```python
from build123d import *

# Parameters (mm, degrees)
F0_R        = 2
F1_DEPTH    = 3.175
F2_R        = 5
F3_R        = 2
F4_W        = 3
F4_H        = 26
F5_DEPTH    = 1
F6_T1_DEPTH = 26


# Not quite as in the source:
# - a fillet or chamfer that OpenCascade refuses, or shapes differently, is made with other operations: its cross-section is extruded or revolved along the edge and cut away or added


with BuildPart() as f1:
    # F0 (on Top) → F1 (new body)
    with BuildSketch(Plane.XY):
        with BuildLine():
            Line((11.2449979984, 0), (0, 0))
            Line((0, 0), (0, 11.2449979984))
            ThreePointArc((0, 11.2449979984), (-0.6568542495, -0.6568542495), (11.2449979984, 0))
        make_face()
        Polygon((0, 11.2449979984), (0, 0), (11.2449979984, 0), (41, 0), (70.7550020016, 0), (82, 0), (82, 11.2449979984), (82, 26), (57.1, 26), (57.1, 21), (41, 21), (24.9, 21), (24.9, 26), (0, 26), align=None)
        with Locations((5, 5)):
            Circle(F0_R, mode=Mode.SUBTRACT)
        with Locations((77, 5)):
            Circle(F0_R, mode=Mode.SUBTRACT)
        with BuildLine():
            Line((82, 0), (70.7550020016, 0))
            ThreePointArc((70.7550020016, 0), (82.6568542495, -0.6568542495), (82, 11.2449979984))
            Line((82, 11.2449979984), (82, 0))
        make_face()
    extrude(amount=F1_DEPTH)

    # F2
    f2_edges = [f1.edges().sort_by_distance(p)[0] for p in [
        (11.244998, 0, 1.5875),
        (70.755002, 0, 1.5875),
        (82, 11.244998, 1.5875),
        (0, 11.244998, 1.5875),
    ]]
    fillet(f2_edges, radius=F2_R)

    # F3
    f3_edges = [f1.edges().sort_by_distance(p)[0] for p in [
        (24.9, 21, 1.5875),
        (57.1, 21, 1.5875),
    ]]
    fillet(f3_edges, radius=F3_R)

    # F4 (on face) → F5 (join)
    with BuildSketch(Plane.XY.offset(3.175)):
        with Locations((20.4, 13)):
            Rectangle(F4_W, F4_H)
        with Locations((61.6, 13)):
            Rectangle(F4_W, F4_H)
    extrude(amount=F5_DEPTH)

    # F6: fillet of radius 5 on 4 edges, made by hand

    # F6_s2 → F6_t1 (join)
    with BuildSketch(Plane.XZ.offset(-26)):
        with BuildLine():
            ThreePointArc((15.9, 3.175), (17.4811388301, 3.4315835097), (18.9, 4.175))
            Line((18.9, 4.175), (18.96, 4.095))
            ThreePointArc((18.96, 4.095), (19, 3.675), (19, 3.175))
            Line((19, 3.175), (18.9, 3.075))
            Line((18.9, 3.075), (15.9, 3.075))
            Line((15.9, 3.075), (15.9, 3.175))
        make_face()
        with BuildLine():
            ThreePointArc((24.9, 3.175), (23.3188611699, 3.4315835097), (21.9, 4.175))
            Line((21.9, 4.175), (21.84, 4.095))
            ThreePointArc((21.84, 4.095), (21.8, 3.675), (21.8, 3.175))
            Line((21.8, 3.175), (21.9, 3.075))
            Line((21.9, 3.075), (24.9, 3.075))
            Line((24.9, 3.075), (24.9, 3.175))
        make_face()
        with BuildLine():
            ThreePointArc((57.1, 3.175), (58.6811388301, 3.4315835097), (60.1, 4.175))
            Line((60.1, 4.175), (60.16, 4.095))
            ThreePointArc((60.16, 4.095), (60.2, 3.675), (60.2, 3.175))
            Line((60.2, 3.175), (60.1, 3.075))
            Line((60.1, 3.075), (57.1, 3.075))
            Line((57.1, 3.075), (57.1, 3.175))
        make_face()
        with BuildLine():
            ThreePointArc((66.1, 3.175), (64.5188611699, 3.4315835097), (63.1, 4.175))
            Line((63.1, 4.175), (63.04, 4.095))
            ThreePointArc((63.04, 4.095), (63, 3.675), (63, 3.175))
            Line((63, 3.175), (63.1, 3.075))
            Line((63.1, 3.075), (66.1, 3.075))
            Line((66.1, 3.075), (66.1, 3.175))
        make_face()
    extrude(amount=F6_T1_DEPTH)


solid = f1.part
```
Input: part model. Units: mm. Frame: model coordinates. A direction names the side the tool comes from. Round coordinates to 2 decimals unless told otherwise and drop trailing zeros. Order: outer loops, then holes, each group sorted by start corner. A loop starts at its lowest first (then second) coordinate and runs counter-clockwise, first axis right, second up. Notation, with made-up numbers: (53.25, 33.5) - (77.25, 33.5) arc R24 ccw to (77.25, 51.5) - close; hole circle Ø6 at (17, 57.25). An arc over 180 degrees is marked (long way). Answer in a Markdown table with one row per item.
Item 1: Line query: line 1 (X direction, y = 24.5, z = 2.7); line 2 (X direction, y = 3.75, z = 2.8); line 3 (Y direction, x = 77, z = 1.35). Output: solid intervals per line, ascending.
Model answer:
| item | result |
|---|---|
| line 1 | x = 0 to 24.9, 57.1 to 82 |
| line 2 | x = -2.9 to 3.44, 6.56 to 75.44, 78.56 to 84.9 |
| line 3 | y = -3 to 3, 7 to 26 |
Item 2: Section query B-B (z = 1.1). Return the cut outline in (x, y).
Model answer:
| item | result |
|---|---|
| outline | (-1.15, 10.11) arc R8 ccw to (10.11, -1.15) arc R5 cw to (13.31, 0) - (68.69, 0) arc R5 cw to (71.89, -1.15) arc R8 ccw to (83.15, 10.11) arc R5 cw to (82, 13.31) - (82, 26) - (57.1, 26) - (57.1, 23) arc R2 cw to (55.1, 21) - (26.9, 21) arc R2 cw to (24.9, 23) - (24.9, 26) - (0, 26) - (0, 13.31) arc R5 cw to start; hole circle Ø4 at (5, 5); hole circle Ø4 at (77, 5) |
Item 3: Mould query, pull axis X, two halves, no side actions, for faces 6 (the flat face through (75, 12, 3.175)), 7 (the cylindrical face through (64.54, 13.182, 3.425)), 8 (the flat face through (41, 9, 3.175)). Classes: released by +X, released by -X, zero draft, split by the parting line, or undercut.
Model answer:
| item | result |
|---|---|
| face 6 | zero draft |
| face 7 | released by +X |
| face 8 | undercut |
Item 4: Reachability of faces 1 (the flat face through (6, 12, 3.175)), 2 (the cylindrical face through (25.47, 21.6, 1.61)), 3 (the cylindrical face through (70.4, -0.3, 1.6)), 4 (the flat face through (0, 20, 2)), 5 (the cylindrical face through (82.54, -0.77, 1.57)) from +Z, -Z, +X, -X, +Y, -Y: full face, straight path, thin tool, end or side. Return the list, or none.
Model answer:
| item | result |
|---|---|
| face 1 | +Z, -X, +Y, -Y |
| face 2 | +Z, -Z, +Y |
| face 3 | +Z, -Z, -Y |
| face 4 | +Z, -Z, -X, +Y |
| face 5 | +Z, -Z |
Item 5: Section query C-C (y = 20.25). Return the cut outline in (x, z) (3 decimals), then the cut area to 3 significant figures.
Model answer:
| item | result |
|---|---|
| outline | (0, 0) - (82, 0) - (82, 3.175) - (66.1, 3.175) arc R5 cw to (63.1, 4.175) - (60.1, 4.175) arc R5 cw to (57.1, 3.175) - (24.9, 3.175) arc R5 cw to (21.9, 4.175) - (18.9, 4.175) arc R5 cw to (15.9, 3.175) - (0, 3.175) - close |
| area | 270 mm² |
Item 6: Section query A-A (x = 77). Return the cut outline in (y, z) (3 decimals), then the cut area to 3 significant figures.
Model answer:
| item | result |
|---|---|
| outline | (-3, 0) - (3, 0) - (3, 3.175) - (-3, 3.175) - close; (7, 0) - (26, 0) - (26, 3.175) - (7, 3.175) - close |
| area | 79.4 mm² |
Item 7: Pin query (flat end, axial travel): pin 1 (1.6 mm diameter, centred on y = 19.5, z = 1, fed in from -X); pin 2 (2.5 mm diameter, centred on x = 77, y = 5, fed in from +Z); pin 3 (1.5 mm diameter, centred on y = 10.5, z = 1.5, fed in from +X); pin 4 (5.5 mm diameter, centred on x = 8, y = 13.5, fed in from +Z) (3 decimals). Return the tip coordinate at first contact, or that it passes through.
Model answer:
| item | result |
|---|---|
| pin 1 | stops at x = 0 |
| pin 2 | passes through |
| pin 3 | stops at x = 83.44 |
| pin 4 | stops at z = 3.175 |
Item 8: Section query D-D (x = 6). Return the cut outline in (y, z) (3 decimals).
Model answer:
| item | result |
|---|---|
| outline | (-2.937, 0) - (3.268, 0) - (3.268, 3.175) - (-2.937, 3.175) - close; (6.732, 0) - (26, 0) - (26, 3.175) - (6.732, 3.175) - close |
